Read the model definition and answer for the solid it produces. Units are mm, in the model's axes. A direction names the side the tool comes from. Coordinates: 2 decimals unless noted, no trailing zeros. Write each loop counter-clockwise with the first axis right and the second up, starting at its lowest first coordinate (ties: lowest second). Pieces come first, ordered by that corner, then holes.
from build123d import *

# Parameters (mm, degrees)
BOSS_EXTRUDE1_DEPTH   = 2.5
SKETCH2_R             = 2
CUT_EXTRUDE1_DEPTH    = 2.5
SKETCH3_R             = 5
CUT_EXTRUDE2_DEPTH    = 2.5
F_3_0MM_DOWEL_HOLE2_D = 3


with BuildPart() as part:
    # Sketch1 → Boss-Extrude1 (new body)
    with BuildSketch(Plane.XY):
        with BuildLine():
            Line((0, 7), (33, 7))
            ThreePointArc((33, 7), (44.66919932, 8.739971416), (55.323194976, 13.808510638))
            ThreePointArc((55.323194976, 13.808510638), (57.187644216, 14.695505002), (59.229754097, 15))
            Line((59.229754097, 15), (68, 15))
            ThreePointArc((68, 15), (72.949747468, 12.949747468), (75, 8))
            Line((75, 8), (75, 0))
            ThreePointArc((75, 0), (72.949747468, -4.949747468), (68, -7))
            Line((68, -7), (0, -7))
            ThreePointArc((0, -7), (-7, 0), (0, 7))
        make_face()
    extrude(amount=BOSS_EXTRUDE1_DEPTH)

    # Sketch2 → Cut-Extrude1 (cut)
    with BuildSketch(Plane.XY.offset(2.5)):
        Circle(SKETCH2_R)
        with Locations((8, 0)):
            Circle(SKETCH2_R)
        with Locations((16, 0)):
            Circle(SKETCH2_R)
    extrude(amount=-CUT_EXTRUDE1_DEPTH, mode=Mode.SUBTRACT)

    # Sketch3 → Cut-Extrude2 (cut)
    with BuildSketch(Plane.XY.offset(2.5)):
        with Locations((64, 4)):
            Circle(SKETCH3_R)
    extrude(amount=-CUT_EXTRUDE2_DEPTH, mode=Mode.SUBTRACT)

    # Ø3.0mm Dowel Hole2 (through all)
    with Locations(Plane.XY.offset(2.5)):
        with Locations((29, -3), (37, -3), (37, 3)):
            Hole(F_3_0MM_DOWEL_HOLE2_D / 2)


solid = part.part
Item 1: Determine the mould class of faces 1 (the cylindrical face through (6, 0, 1)), 2 (the cylindrical face through (-7, 0, 1)), 3 (the flat face through (34, -7, 1)) for opening direction X: +X half, -X half, draft (parallel to the pull), parting line (faces both ways), or undercut.
Item 2: For faces 4 (the flat face through (16, 7, 1)), 5 (the cylindrical face through (14.4, -1.2, 1.3)), determine the directions among +Z, -Z, +X, -X, +Y, -Y from which every point of the face is accessible in a straight line to the end or side of a thin tool.
Item 3: The part is cut by section A-A (x = 64). Give the vertices of the cut face in (y, z).
Item 4: The part is cut by section C-C (z = 0.75). Give the vertices of the cut face in (x, y).
Item 5: The part is cut by section B-B (y = -3). Give the vertices of the cut face in (x, z), and give its area (3 significant figures).
Item 6: Find the intervals of material crossed by probe 1 along Y at (x, z) = (0, 1.45); probe 2 along X at (y, z) = (1.25, 2.2); probe 3 along X at (y, z) = (4.25, 0.2), in increasing order.
Item 7: Given pin 1 (3 mm diameter, centred on x = 0, y = 0, fed in from -Z); pin 2 (1 mm diameter, centred on x = 12, z = 1.5, fed in from +Y); pin 3 (1 mm diameter, centred on y = -3, z = 1.5, fed in from +X), each flat-ended and moving along its own axis, determine where each tip first touches the part or whether it passes through.
Item 8: The part is cut by section D-D (x = 37). Give the vertices of the cut face in (y, z), and give its area (3 significant figures).
Answer:
1. face 1: undercut
1. face 2: -X half
1. face 3: draft
2. face 4: +Z, -Z, -X, +Y
2. face 5: +Z, -Z
3. outline: (-7, 0) - (-1, 0) - (-1, 2.5) - (-7, 2.5) - close; (9, 0) - (15, 0) - (15, 2.5) - (9, 2.5) - close
4. outline: (0, -7) - (68, -7) arc R7 ccw to (75, 0) - (75, 8) arc R7 ccw to (68, 15) - (59.23, 15) arc R7 ccw to (55.32, 13.81) arc R40 cw to (33, 7) - (0, 7) arc R7 ccw to start; hole circle Ø4 at (0, 0); hole circle Ø4 at (8, 0); hole circle Ø4 at (16, 0); hole circle Ø3 at (29, -3); hole circle Ø3 at (37, -3); hole circle Ø3 at (37, 3); hole circle Ø10 at (64, 4)
5. outline: (-6.32, 0) - (27.5, 0) - (27.5, 2.5) - (-6.32, 2.5) - close; (30.5, 0) - (35.5, 0) - (35.5, 2.5) - (30.5, 2.5) - close; (38.5, 0) - (74.32, 0) - (74.32, 2.5) - (38.5, 2.5) - close
5. area: 187 mm2
6. probe 1: y = -7 to -2, 2 to 7
6. probe 2: x = -6.89 to -1.56, 1.56 to 6.44, 9.56 to 14.44, 17.56 to 59.82, 68.18 to 75
6. probe 3: x = -5.56 to 36.17, 37.83 to 59.01, 68.99 to 75
7. pin 1: passes through
7. pin 2: stops at y = 7
7. pin 3: stops at x = 74.54
8. outline: (-7, 0) - (-4.5, 0) - (-4.5, 2.5) - (-7, 2.5) - close; (-1.5, 0) - (1.5, 0) - (1.5, 2.5) - (-1.5, 2.5) - close; (4.5, 0) - (7.2, 0) - (7.2, 2.5) - (4.5, 2.5) - close
8. area: 20.5 mm2
